Here's the drawing with two shaded views (mm, measured from the low corner). I have some questions. A direction names the side the tool comes from. Coordinates: 2 decimals unless noted, no trailing zeros. Write each loop counter-clockwise with the first axis right and the second up, starting at its lowest first coordinate (ties: lowest second). Pieces come first, ordered by that corner, then holes.
Item 1: If we section it at B-B (z = 66): Please give me the cut outline in (x, y).
Item 2: I'm going to push flat-ended pins straight in: pin 1 Ø6 at (x, y) = (48, 7) entering from -Z; pin 2 Ø3.5 at (x, z) = (68, 36) entering from +Y; pin 3 Ø10 at (y, z) = (26.5, 24.5) entering from -X. Where does each tip first touch, or does it pass through?
Item 3: If we section it at A-A (x = 6): Please give me the cut outline in (y, z), then the cut area to 3 significant figures.
Item 4: For the marked faces 1 and 2, which set-ups out of +Z, -Z, +X, -X, +Y, -Y let a thin tool reach every point of the face, with its end or its side?
Item 5: If we section it at D-D (z = 15): Please give me the cut outline in (x, y).
Item 6: If we section it at C-C (x = 20): Please give me the cut outline in (y, z), then the cut area to 3 significant figures.
Item 7: If I drill on line 1 (X direction, y = 1.4, z = 5); line 2 (X direction, y = 1.65, z = 36); line 3 (Y direction, x = 37, z = 20), over which ranges is the centre line in solid material (lowest first)?
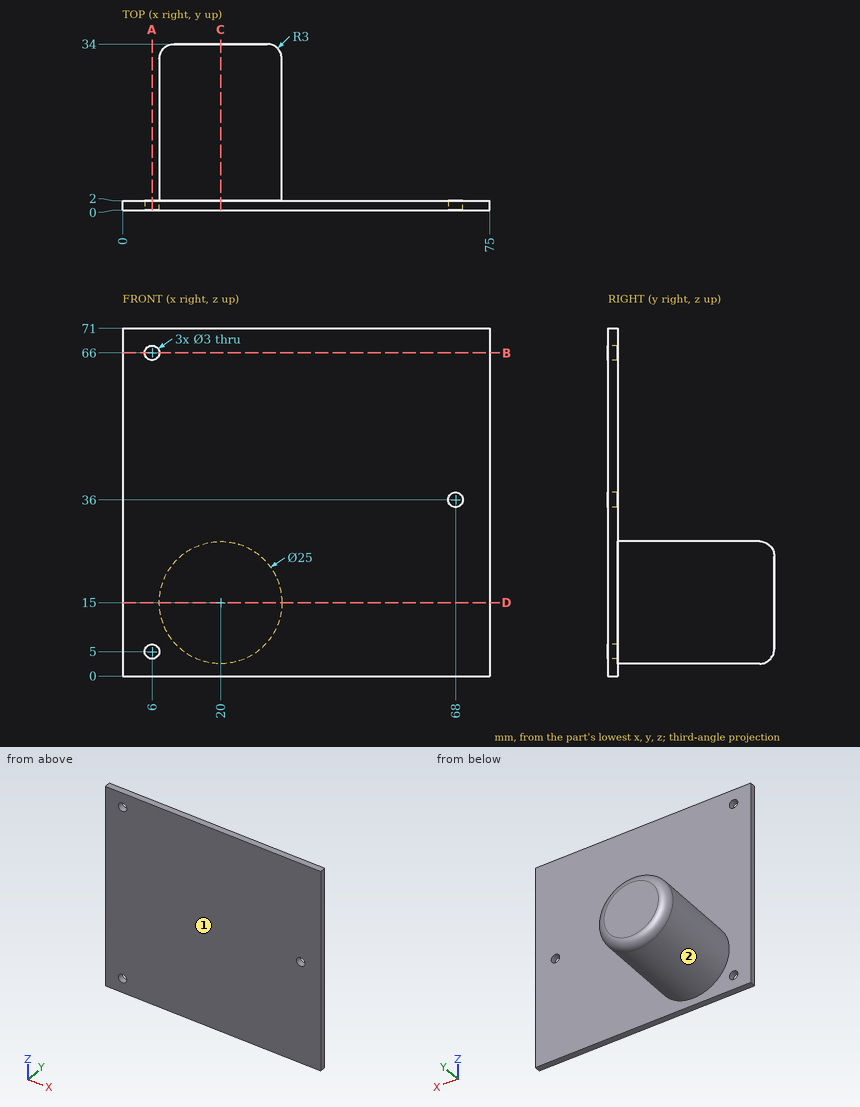
Answer list:
1. outline: (0, 0) - (4.5, 0) - (4.5, 2) - (0, 2) - close; (7.5, 0) - (75, 0) - (75, 2) - (7.5, 2) - close
2. pin 1: passes through
2. pin 2: stops at y = 2
2. pin 3: stops at x = 8.34
3. outline: (0, 0) - (2, 0) - (2, 3.5) - (0, 3.5) - close; (0, 6.5) - (2, 6.5) - (2, 64.5) - (0, 64.5) - close; (0, 67.5) - (2, 67.5) - (2, 71) - (0, 71) - close
3. area: 130 mm2
4. face 1: +Z, -Z, +X, -X, -Y
4. face 2: +Y
5. outline: (0, 0) - (75, 0) - (75, 2) - (32.5, 2) - (32.5, 31) arc R3 ccw to (29.5, 34) - (10.5, 34) arc R3 ccw to (7.5, 31) - (7.5, 2) - (0, 2) - close
6. outline: (0, 0) - (2, 0) - (2, 2.5) - (31, 2.5) arc R3 ccw to (34, 5.5) - (34, 24.5) arc R3 ccw to (31, 27.5) - (2, 27.5) - (2, 71) - (0, 71) - close
6. area: 938 mm2
7. line 1: x = 0 to 4.5, 7.5 to 75
7. line 2: x = 0 to 66.5, 69.5 to 75
7. line 3: y = 0 to 2
